Can you work these out from the drawing? Everything is in mm from the part's minimum corner. Give positions to 0.01 mm unless a question says otherwise; leave off trailing zeros. Loops run counter-clockwise (first coordinate to the right, second up) from the corner with the lowest first, then second, coordinate; pieces in that order, holes last. Notation, with made-up numbers: M 22.25,-28 L 78.25,-28 A25 ccw 78.25,-14 Z; hole C -31,-36.5 d11. An arc over 180 degrees is marked long. Use CSV: the item, a comma, the result in double quotes.
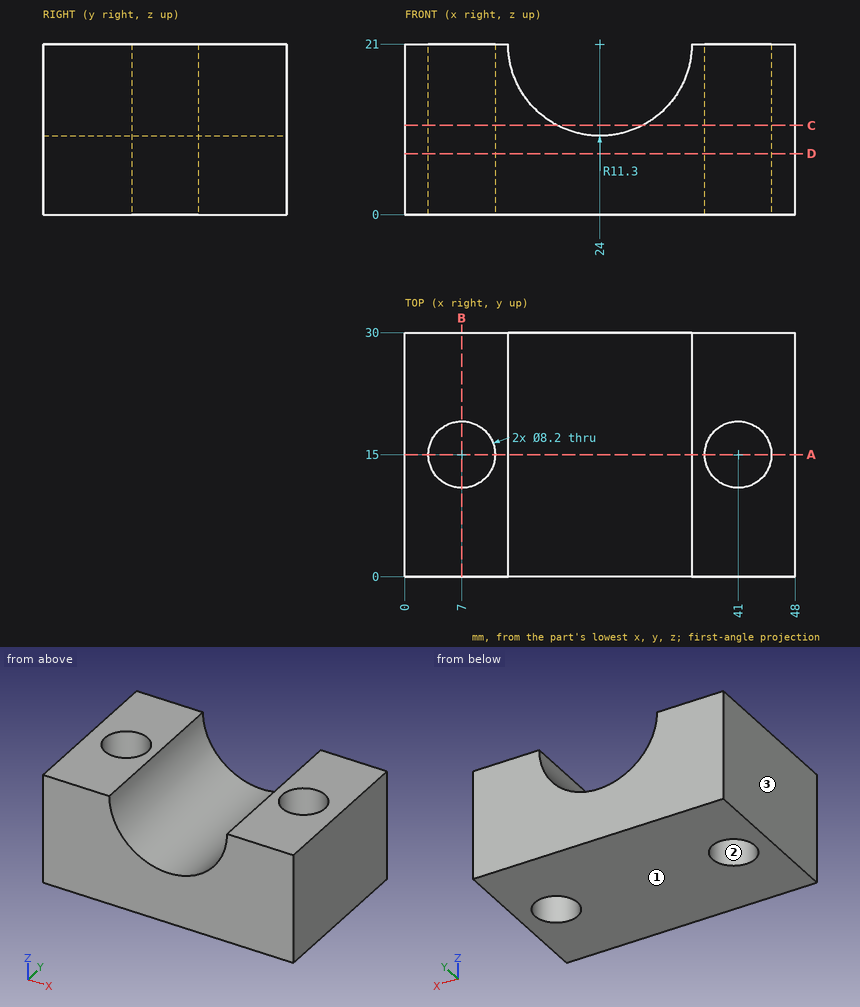
Q1. I want a section at B-B, the plane x = 7. Please give me the cut outline in (y, z), then the cut area to 3 significant figures.
Model answer:
outline,"M 0,0 L 10.9,0 L 10.9,21 L 0,21 Z; M 19.1,0 L 30,0 L 30,21 L 19.1,21 Z"
area,"458 mm2"
Q2. I'm going to push a flat-ended pin straight in: P1, Ø1.5, axis at x = 29, y = 24.5, coming from the +Z side. Where does the tip first touch, or does it pass through?
Model answer:
P1,"z = 11.27"
Q3. I want a section at C-C, the plane z = 11. Please give me the cut outline in (x, y), then the cut area to 3 significant figures.
Model answer:
outline,"M 0,0 L 18.74,0 L 18.74,30 L 0,30 Z; M 29.26,0 L 48,0 L 48,30 L 29.26,30 Z; hole C 7,15 d8.2; hole C 41,15 d8.2"
area,"1,020 mm2"
Q4. If we mould it in two halves opening along X, with no side actions, what happens to the marked faces 1, 2 and 3? For each: released by +X, released by -X, zero draft, split by the parting line, or undercut.
Model answer:
face 1,"zero draft"
face 2,"undercut"
face 3,"released by -X"
Q5. I want a section at A-A, the plane y = 15. Please give me the cut outline in (x, z).
Model answer:
outline,"M 0,0 L 2.9,0 L 2.9,21 L 0,21 Z; M 11.1,0 L 36.9,0 L 36.9,21 L 35.3,21 A11.3 cw 12.7,21 L 11.1,21 Z; M 45.1,0 L 48,0 L 48,21 L 45.1,21 Z"
Q6. I want a section at D-D, the plane z = 7.5. Please give me the cut outline in (x, y), then the cut area to 3 significant figures.
Model answer:
outline,"M 0,0 L 48,0 L 48,30 L 0,30 Z; hole C 7,15 d8.2; hole C 41,15 d8.2"
area,"1,330 mm2"
Q7. Please list where these lines run through material, in increasing order: L1, parallel to Y at x = 41, z = 14.5; L2, parallel to X at y = 11.25, z = 15.25; L3, parallel to X at y = 12, z = 18.5. Write a range as from..to.
Model answer:
L1,"0..10.9, 19.1..30"
L2,"0..5.34, 8.66..14.27, 33.73..39.34, 42.66..48"
L3,"0..4.21, 9.79..12.98, 35.02..38.21, 43.79..48"
